from build123d import *

# Parameters (mm, degrees)
EXTRUDE_1_DEPTH     = 8
SKETCH_2_R          = 6.1
CUT_EXTRUDE_1_DEPTH = 93
SKETCH_4_R          = 12.5
CUT_EXTRUDE_3_DEPTH = 93
SKETCH_5_R          = 2.6
CUT_EXTRUDE_4_DEPTH = 93
SKETCH_6_R          = 5.5
CUT_EXTRUDE_5_DEPTH = 1.5


with BuildPart() as part:
    # 草图1 → 凸台-拉伸1 (new body)
    with BuildSketch(Plane(origin=(0, 0, 0), x_dir=(1, 0, 0), z_dir=(0, 1, 0))):
        Polygon((69.282032303, 0), (34.641016151, 60), (-34.641016151, 60), (-69.282032303, 0), (-34.641016151, -60), (34.641016151, -60), align=None)
    extrude(amount=EXTRUDE_1_DEPTH)

    # 草图2 → 切除-拉伸1 (cut, through all)
    with BuildSketch(Plane(origin=(0, 8, 0), x_dir=(1, 0, 0), z_dir=(0, 1, 0))):
        with Locations(Location((-50, 0, 0), (0, 0, 270))):
            Circle(SKETCH_2_R)
        with Locations(Location((50, 0, 0), (0, 0, 270))):
            Circle(SKETCH_2_R)
    extrude(amount=-CUT_EXTRUDE_1_DEPTH, mode=Mode.SUBTRACT)

    # 草图4 → 切除-拉伸3 (cut, through all)
    with BuildSketch(Plane(origin=(0, 8, 0), x_dir=(1, 0, 0), z_dir=(0, 1, 0))):
        with Locations(Location((0, 0, 0), (0, 0, 270))):
            Circle(SKETCH_4_R)
    extrude(amount=-CUT_EXTRUDE_3_DEPTH, mode=Mode.SUBTRACT)

    # 草图5 → 切除-拉伸4 (cut, through all)
    with BuildSketch(Plane(origin=(0, 8, 0), x_dir=(1, 0, 0), z_dir=(0, 1, 0))):
        with Locations(Location((-10, -28.284271247, 0), (0, 0, 270))):
            Circle(SKETCH_5_R)
        with Locations(Location((-19.494897428, 22.802389662, 0), (0, 0, 270))):
            Circle(SKETCH_5_R)
        with Locations(Location((29.494897428, 5.481881586, 0), (0, 0, 270))):
            Circle(SKETCH_5_R)
    extrude(amount=-CUT_EXTRUDE_4_DEPTH, mode=Mode.SUBTRACT)

    # 草图6 → 切除-拉伸5 (cut)
    with BuildSketch(Plane.XZ):
        with Locations(Location((-10, 28.284271247, 0), (0, 0, 270))):
            Circle(SKETCH_6_R)
        with Locations(Location((-19.494897428, -22.802389662, 0), (0, 0, 270))):
            Circle(SKETCH_6_R)
        with Locations(Location((29.494897428, -5.481881586, 0), (0, 0, 270))):
            Circle(SKETCH_6_R)
    extrude(amount=-CUT_EXTRUDE_5_DEPTH, mode=Mode.SUBTRACT)


solid = part.part
Build history of the part. All positions in model axes, mm. A direction names the side the tool comes from. Give positions to 0.01 mm unless a question says otherwise; leave off trailing zeros. Loops run counter-clockwise (first coordinate to the right, second up) from the corner with the lowest first, then second, coordinate; pieces in that order, holes last. Notation, with made-up numbers: (37, -9) -> (62, -9) arc R14 ccw to (62, 12) -> close; hole circle Ø3 at (-6, 72.25). An arc over 180 degrees is marked (long way). Answer in a Markdown table with one row per item.
Item 1: Flat gauge pins, fed straight in: P1, Ø4, axis at y = 4.5, z = 32.5, coming from the +X side; P2, Ø2, axis at x = -37, y = 4.5, coming from the -Z side; P3, Ø12.5, axis at x = -19.49, z = -22.8, coming from the -Y side; P4, Ø22.5, axis at x = 0, z = 0, coming from the +Y side. Where does each tip first touch, or does it go through?
Findings below:
| item | result |
|---|---|
| P1 | stops at x = 51.67 |
| P2 | stops at z = -57.65 |
| P3 | stops at y = 0 |
| P4 | passes through |
Item 2: Slice it at A-A on x = -10. Write the cut outline in (y, z).
Findings below:
| item | result |
|---|---|
| outline | (0, -60) -> (8, -60) -> (8, -7.5) -> (0, -7.5) -> close; (0, 7.5) -> (8, 7.5) -> (8, 25.68) -> (1.5, 25.68) -> (1.5, 22.78) -> (0, 22.78) -> close; (0, 33.78) -> (1.5, 33.78) -> (1.5, 30.88) -> (8, 30.88) -> (8, 60) -> (0, 60) -> close |
Item 3: Probe line 1 along X through (y, z) = (3.5, 0); line 2 along X through (y, z) = (5, 4); line 3 along X through (y, z) = (0.5, 27.5). List the from-to ranges inside material, lowest first. Write a range as [from, to].
Findings below:
| item | result |
|---|---|
| line 1 | x = [-69.28, -56.1], [-43.9, -12.5], [12.5, 43.9], [56.1, 69.28] |
| line 2 | x = [-66.97, -54.61], [-45.39, -11.84], [11.84, 45.39], [54.61, 66.97] |
| line 3 | x = [-53.4, -15.44], [-4.56, 53.4] |
Item 4: Slice it at C-C on y = 6.75. Write the cut outline in (x, z).
Findings below:
| item | result |
|---|---|
| outline | (-69.28, 0) -> (-34.64, -60) -> (34.64, -60) -> (69.28, 0) -> (34.64, 60) -> (-34.64, 60) -> close; hole circle Ø12.2 at (-50, 0); hole circle Ø5.2 at (-19.49, -22.8); hole circle Ø5.2 at (-10, 28.28); hole circle Ø25 at (0, 0); hole circle Ø5.2 at (29.49, -5.48); hole circle Ø12.2 at (50, 0) |
Item 5: Mould opens along X. For faces 3 (the flat face through (-52.204, 3.944, 29.58)), 4 (the cylindrical face through (-24.864, 0.74, -21.61)), 5 (the flat face through (0, 4, 60)) say: pulls with the +X half, pulls with the -X half, needs draft (parallel to the pull), parting line crosses it, or undercut.
Findings below:
| item | result |
|---|---|
| face 3 | pulls with the -X half |
| face 4 | undercut |
| face 5 | needs draft |
Item 6: Slice it at D-D on z = 49.5. Write the cut outline in (x, y).
Findings below:
| item | result |
|---|---|
| outline | (-40.7, 0) -> (40.7, 0) -> (40.7, 8) -> (-40.7, 8) -> close |
Item 7: Tool access for faces 1 (the flat face through (0, 4, -60)), 2 (the flat face through (-11, 1.5, 31)): list every direction of +Z, -Z, +X, -X, +Y, -Y with a clear straight run to the whole face (end or side of a thin tool).
Findings below:
| item | result |
|---|---|
| face 1 | -Z, +X, -X, +Y, -Y |
| face 2 | -Y |
Item 8: Slice it at B-B on x = -50. Write the cut outline in (y, z), plus the area to 3 significant figures.
Findings below:
| item | result |
|---|---|
| outline | (0, -33.4) -> (8, -33.4) -> (8, -6.1) -> (0, -6.1) -> close; (0, 6.1) -> (8, 6.1) -> (8, 33.4) -> (0, 33.4) -> close |
| area | 437 mm² |
